Could you check a few things on this drawing? It's one solid part, dimensions in mm from its lowest x, y, z. A direction names the side the tool comes from. Give positions to 0.01 mm unless a question says otherwise; leave off trailing zeros. Order: outer loops, then holes, each group sorted by start corner. A loop starts at its lowest first (then second) coordinate and runs counter-clockwise, first axis right, second up. Notation, with made-up numbers: (43.25, 83.25) - (50.25, 83.25) arc R17 cw to (50.25, 112.25) - close; hole circle Ø8 at (49, 1). An arc over 180 degrees is marked (long way). One line per question, with ' | ' between items. Start each with the question number.
1. Imagine slicing it at B-B (y = 20). Please give me the cut outline in (x, z).
2. Imagine slicing it at C-C (x = 8). Please give me the cut outline in (y, z), and give its area (3 significant figures).
3. Which directions (+Z, -Z, +X, -X, +Y, -Y) give clear straight access to the entire face, cutting with the end or side of a thin tool? Please do the marked faces 1, 2, 3 and 4.
4. I need wall thicknesses on probe 1 along X at (y, z) = (6, 14.5); probe 2 along X at (y, z) = (28, 9.5); probe 3 along Y at (x, z) = (114, 8.75). Which ranges of each line are inside material? Lowest first, please. Write a range as from..to.
5. Imagine slicing it at A-A (z = 14.25). Please give me the cut outline in (x, y), and give its area (3 significant figures).
6. For P1, Ø4.5, axis at y = 42, z = 7.5, coming from the -X side; P2, Ø4.5, axis at y = 5, z = 15.5, coming from the +X side; P3, Ø4, axis at x = 43.5, y = 21.5, coming from the -Z side, each with a flat end and sliding along its axis, tell me the tip position at first contact or that it passes through.
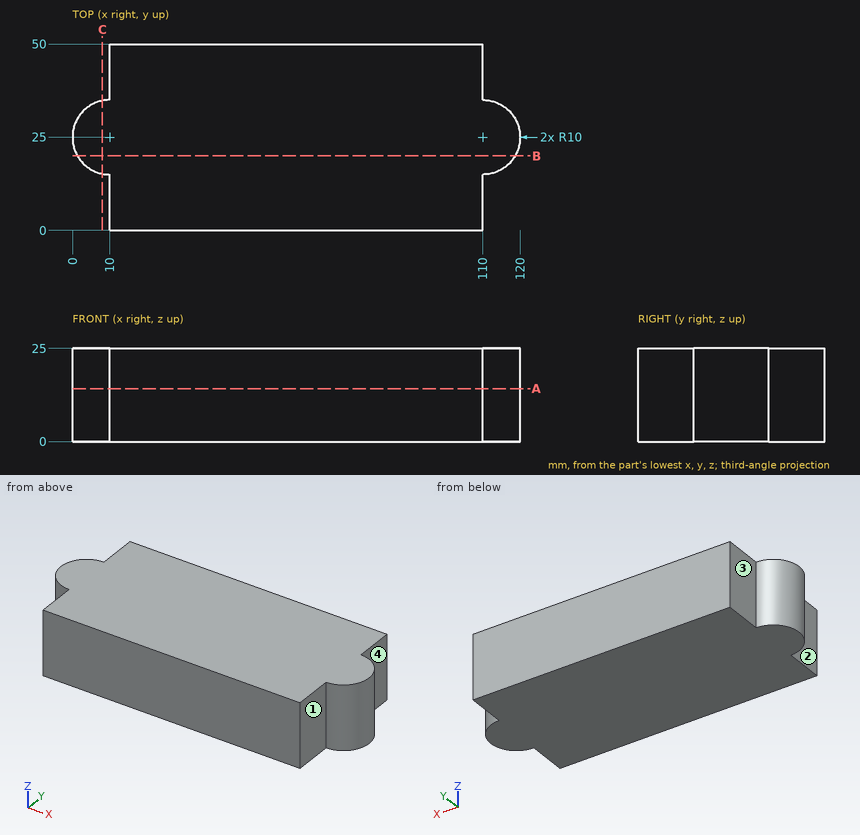
Results found:
1) outline: (1.34, 0) - (118.66, 0) - (118.66, 25) - (1.34, 25) - close
2) outline: (15.2, 0) - (34.8, 0) - (34.8, 25) - (15.2, 25) - close | area: 490 mm2
3) face 1: +Z, -Z, +X, -Y | face 2: +Z, -Z, -X, -Y | face 3: +Z, -Z, -X, +Y | face 4: +Z, -Z, +X, +Y
4) probe 1: x = 10..110 | probe 2: x = 0.46..119.54 | probe 3: y = 15.83..34.17
5) outline: (10, 0) - (110, 0) - (110, 15) arc R10 ccw to (110, 35) - (110, 50) - (10, 50) - (10, 35) arc R10 ccw to (10, 15) - close | area: 5,310 mm2
6) P1: stops at x = 10 | P2: stops at x = 110 | P3: stops at z = 0
